from build123d import *

# Parameters (mm, degrees)
SKETCH1_W         = 9.652
SKETCH1_H         = 4.5
BUTTON_BASE_DEPTH = 3.556
SKETCH2_W         = 10.9020356
SKETCH2_H         = 5.7500356
GUIDE_DEPTH       = 1
SKETCH3_R         = 2.54
ARM_DEPTH         = 1.6002
CHAMFER1_SIZE     = 0.375
FILLET1_R         = 0.25
FILLET2_R         = 0.254


with BuildPart() as part:
    # Sketch1 → Button Base (new body)
    with BuildSketch(Plane.XY):
        Rectangle(SKETCH1_W, SKETCH1_H)
    extrude(amount=BUTTON_BASE_DEPTH)

    # Sketch2 → Guide (add)
    with BuildSketch(Plane(origin=(0, 0, 0), x_dir=(-1, 0, 0), z_dir=(0, 0, -1))):
        Rectangle(SKETCH2_W, SKETCH2_H)
    extrude(amount=GUIDE_DEPTH)

    # Sketch3 → Arm (add)
    with BuildSketch(Plane(origin=(0, 0, -1), x_dir=(-1, 0, 0), z_dir=(0, 0, -1))):
        Circle(SKETCH3_R)
    extrude(amount=ARM_DEPTH)

    # Chamfer1
    chamfer1_edges = [part.edges().sort_by_distance(p)[0] for p in [
        (0, -2.8750178, 0),
        (-5.4510178, 0, 0),
        (0, 2.8750178, 0),
        (5.4510178, 0, 0),
    ]]
    chamfer(chamfer1_edges, length=CHAMFER1_SIZE)

    # Fillet1
    fillet1_edges = [part.edges().sort_by_distance(p)[0] for p in [
        (5.4510178, -2.8750178, -0.6875),
        (-5.4510178, -2.8750178, -0.6875),
        (-5.4510178, 2.8750178, -0.6875),
        (5.4510178, 2.8750178, -0.6875),
    ]]
    fillet(fillet1_edges, radius=FILLET1_R)

    # Fillet2
    fillet2_edges = [part.edges().sort_by_distance(p)[0] for p in [
        (2.54, 0, -2.6002),
    ]]
    fillet(fillet2_edges, radius=FILLET2_R)


solid = part.part
Can you work these out from the model? Positions are in its coordinate system, mm. A direction names the side the tool comes from. Round coordinates to 2 decimals unless told otherwise and drop trailing zeros. Loops run counter-clockwise (first coordinate to the right, second up) from the corner with the lowest first, then second, coordinate; pieces in that order, holes last. Notation, with made-up numbers: (62, -25.75) - (71, -25.75) arc R16 cw to (71, -6.75) - close; hole circle Ø7 at (1.5, 75.25). An arc over 180 degrees is marked (long way). Write item = value, one per line. Start each with the question number.
(1) For P1, Ø1.8, axis at y = -0.5, z = 1.5, coming from the +X side; P2, Ø1.8, axis at x = -1, z = 2.5, coming from the +Y side, each with a flat end and sliding along its axis, tell me the tip position at first contact or that it passes through.
(2) If we section it at C-C (z = -1.5): Please give me the cut outline in (x, y), and give its area (3 significant figures).
(3) If we section it at A-A (y = 0): Please give me the cut outline in (x, z) (3 decimals).
(4) If I drill on probe 1 along Z at (x, y) = (1.25, 2.15); probe 2 along Z at (x, y) = (-4.25, -0.8); probe 3 along X at (y, z) = (0.25, 1.25), over which ranges is the centre line in solid material (lowest first)? Write a range as [from, to].
(5) If we section it at D-D (x = 0): Please give me the cut outline in (y, z) (3 decimals).
(6) If we section it at B-B (x = 3.75): Please give me the cut outline in (y, z) (3 decimals).
(7) For faces 1 (the face through (0, -2.25, 2)), 2 (the face through (-4.826, 0, 2)), 3 (the face through (0, 2.25, 2)), 4 (the face through (0.33, 2.52, -1.66)), 5 (the face through (4.826, 0, 2)), which set-ups out of +Z, -Z, +X, -X, +Y, -Y let a thin tool reach every point of the face, with its end or its side?
Ans:
q1.P1 = 4.83
q1.P2 = 2.25
q2.outline = circle Ø5.08 at (0, 0)
q2.area = 20.3 mm²
q3.outline = (-5.451, -1) - (-2.54, -1) - (-2.54, -2.346) arc R0.254 ccw to (-2.286, -2.6) - (2.286, -2.6) arc R0.254 ccw to (2.54, -2.346) - (2.54, -1) - (5.451, -1) - (5.451, -0.375) - (5.076, 0) - (4.826, 0) - (4.826, 3.556) - (-4.826, 3.556) - (-4.826, 0) - (-5.076, 0) - (-5.451, -0.375) - close
q4.probe_1 = [-2.5, 3.56]
q4.probe_2 = [-1, 3.56]
q4.probe_3 = [-4.83, 4.83]
q5.outline = (-2.875, -1) - (-2.54, -1) - (-2.54, -2.346) arc R0.254 ccw to (-2.286, -2.6) - (2.286, -2.6) arc R0.254 ccw to (2.54, -2.346) - (2.54, -1) - (2.875, -1) - (2.875, -0.375) - (2.5, 0) - (2.25, 0) - (2.25, 3.556) - (-2.25, 3.556) - (-2.25, 0) - (-2.5, 0) - (-2.875, -0.375) - close
q6.outline = (-2.875, -1) - (2.875, -1) - (2.875, -0.375) - (2.5, 0) - (2.25, 0) - (2.25, 3.556) - (-2.25, 3.556) - (-2.25, 0) - (-2.5, 0) - (-2.875, -0.375) - close
q7.face_1 = +Z, +X, -X, -Y
q7.face_2 = +Z, -X, +Y, -Y
q7.face_3 = +Z, +X, -X, +Y
q7.face_4 = -Z
q7.face_5 = +Z, +X, +Y, -Y
